from build123d import *

# Parameters (mm, degrees)
EXTRUDE_1_DEPTH        = 9
SKETCH_3_R             = 15
CUT_EXTRUDE_1_DEPTH    = 26.5
HOLE_WIZARD_M6_1_D     = 5
HOLE_WIZARD_M6_1_DEPTH = 17
HOLE_WIZARD_M6_1_TIP   = 1.502151548
CHAMFER_1_SIZE         = 1
SKETCH_6_W             = 1.1
SKETCH_6_H             = 0.3


with BuildPart() as part:
    # 草图1 → 旋转1 (revolve)
    with BuildSketch(Plane.XY, mode=Mode.PRIVATE) as revolve_1_sk:
        Polygon((-89.5, 0), (89.5, 0), (89.5, 6), (88.5, 7), (-6, 7), (-6, 10), (-8.5, 10), (-8.5, 7), (-89, 7), (-89.5, 6.5), align=None)
    revolve(revolve_1_sk.sketch.rotate(Axis((-89.5, 0, 0), (1, 0, 0)), 90), axis=Axis((-89.5, 0, 0), (1, 0, 0)))

    # 草图2 → 凸台-拉伸1 (add)
    with BuildSketch(Plane.XY):
        with BuildLine():
            Line((68.5, -2.5), (83.5, -2.5))
            ThreePointArc((83.5, -2.5), (86, 0), (83.5, 2.5))
            Line((83.5, 2.5), (68.5, 2.5))
            ThreePointArc((68.5, 2.5), (66, 0), (68.5, -2.5))
        make_face()
        with BuildLine():
            ThreePointArc((-83.5, 2.5), (-86, 0), (-83.5, -2.5))
            Line((-83.5, -2.5), (-68.5, -2.5))
            ThreePointArc((-68.5, -2.5), (-66, 0), (-68.5, 2.5))
            Line((-68.5, 2.5), (-83.5, 2.5))
        make_face()
        with BuildLine():
            Line((1, 2.5), (-1, 2.5))
            ThreePointArc((-1, 2.5), (-3.5, 0), (-1, -2.5))
            Line((-1, -2.5), (1, -2.5))
            ThreePointArc((1, -2.5), (3.5, 0), (1, 2.5))
        make_face()
        with BuildLine():
            Line((52, 2.5), (42, 2.5))
            ThreePointArc((42, 2.5), (39.5, 0), (42, -2.5))
            Line((42, -2.5), (52, -2.5))
            ThreePointArc((52, -2.5), (54.5, 0), (52, 2.5))
        make_face()
    extrude(amount=EXTRUDE_1_DEPTH)

    # 草图3 → 切除-拉伸1 (cut)
    with BuildSketch(Plane(origin=(89.5, 0, 0), x_dir=(0, 0, -1), z_dir=(1, 0, 0))):
        Circle(SKETCH_3_R)
    extrude(amount=-CUT_EXTRUDE_1_DEPTH, mode=Mode.SUBTRACT)

    # M6 螺纹孔1
    with Locations(Plane.ZY.offset(89.5)):
        with Locations((0, 0)):
            Hole(HOLE_WIZARD_M6_1_D / 2, depth=HOLE_WIZARD_M6_1_DEPTH)
            with Locations((0, 0, -(HOLE_WIZARD_M6_1_DEPTH + HOLE_WIZARD_M6_1_TIP / 2))):  # 118° drill point
                Cone(0, HOLE_WIZARD_M6_1_D / 2, HOLE_WIZARD_M6_1_TIP, mode=Mode.SUBTRACT)

    # 倒角1
    chamfer_1_edges = [part.edges().sort_by_distance(p)[0] for p in [
        (63, 0, -7),
    ]]
    chamfer(chamfer_1_edges, length=CHAMFER_1_SIZE)

    # 草图6 → 切除-旋转1 (revolve, cut)
    with BuildSketch(Plane.XY, mode=Mode.PRIVATE) as cut_revolve_1_sk:
        with Locations((57.55, -6.85)):
            Rectangle(SKETCH_6_W, SKETCH_6_H)
    revolve(cut_revolve_1_sk.sketch.rotate(Axis((0, 0, 0), (1, 0, 0)), 270), axis=Axis((0, 0, 0), (1, 0, 0)), mode=Mode.SUBTRACT)


solid = part.part
Check sheet for the modelled part. Datum: model origin and axes. Units: mm. A direction names the side the tool comes from. Round coordinates to 2 decimals unless told otherwise and drop trailing zeros. Write each loop counter-clockwise with the first axis right and the second up, starting at its lowest first coordinate (ties: lowest second). Pieces come first, ordered by that corner, then holes. Notation, with made-up numbers: (85, 28) -> (101, 28) arc R35 cw to (101, 65) -> close; hole circle Ø2 at (67.25, 41.5). An arc over 180 degrees is marked (long way). Answer as CSV lines item,"result". Start each with the question number.
1) Material ranges on line 1 (Z direction, x = -84, y = 0); line 2 (Y direction, x = -79.25, z = 0); line 3 (X direction, y = 1, z = -2.25), recorded low to high. Write a range as from..to.
2) Section check A-A on x = -76. Enter the section's corners in (y, z).
3) Tool access check on faces 5 (the cylindrical face through (-3.5, 0.1, 7.8)), 6 (the flat face through (47, 0, 9)), 7 (the flat face through (-76, -2.5, 8)), 8 (the flat face through (47, 2.5, 8)), 9 (the cylindrical face through (-86, 0, 8)). Record the directions out of +Z, -Z, +X, -X, +Y, -Y that give a thin tool (end or side, any length) a straight path to the whole face; none if there is none.
4) Release check for a two-part mould opening along X. For faces 1 (the cylindrical face through (57.558, -0.295, -6.694)), 2 (the cylindrical face through (-7, 0, -10)), 3 (the cylindrical face through (54.5, -0.1, 7.8)), 4 (the conical face through (-71, 0, 0)) record: pulls with the +X half, pulls with the -X half, needs draft (parallel to the pull), parting line crosses it, or undercut.
5) Go/stop test with flat-tipped pins: P1, Ø2.5, axis at x = -77.5, z = 7.5, coming from the -Y side; P2, Ø12, axis at x = -25, z = 6, coming from the +Y side; P3, Ø1.5, axis at x = 37, y = 2, coming from the -Z side. Record where each tip stops, or that it passes through.
6) Section check C-C on z = -8.25. Enter the section's corners in (x, y).
7) Section check B-B on x = 22. Enter the section's corners in (y, z), and give its area (3 significant figures).
Found:
1,line 1,"z = -7..-2.5, 2.5..9"
1,line 2,"y = -7..-2.5, 2.5..7"
1,line 3,"x = -72.48..63"
2,outline,"(-2.5, 6.54) arc R7 ccw (long way) to (2.5, 6.54) -> (2.5, 9) -> (-2.5, 9) -> close; hole circle Ø5 at (0, 0)"
3,face 5,"+Z"
3,face 6,"+Z, +X, +Y, -Y"
3,face 7,"+Z, -X, -Y"
3,face 8,"+Z, +X, +Y"
3,face 9,"+Z, -X"
4,face 1,"undercut"
4,face 2,"needs draft"
4,face 3,"pulls with the +X half"
4,face 4,"pulls with the -X half"
5,P1,"stops at y = -3.15"
5,P2,"stops at y = 7"
5,P3,"stops at z = -6.89"
6,outline,"(-8.5, -5.65) -> (-6, -5.65) -> (-6, 5.65) -> (-8.5, 5.65) -> close"
7,outline,"circle Ø14 at (0, 0)"
7,area,"154 mm^2"
